Could you check a few things on this model? Use its own coordinates, in mm. A direction names the side the tool comes from. Coordinates: 2 decimals unless noted, no trailing zeros. Order: outer loops, then holes, each group sorted by start corner. A loop starts at its lowest first (then second) coordinate and runs counter-clockwise, first axis right, second up. Notation, with made-up numbers: M 88.25,18.25 L 103.25,18.25 A24 cw 103.25,57.25 Z; hole C 6.5,47.25 d9. An arc over 180 degrees is marked long. Write item = value, one per line. Start each with the question number.
from build123d import *

# Parameters (mm, degrees)
FORO_LAMATO_PER_VITE_M4_A_TESTA_CILINDRI_D           = 4.5
FORO_LAMATO_PER_VITE_M4_A_TESTA_CILINDRI_CBORE_D     = 8
FORO_LAMATO_PER_VITE_M4_A_TESTA_CILINDRI_CBORE_DEPTH = 2.6
RIPETIZIONECIRCOLARE1_COUNT                          = 4
RACCORDO1_R                                          = 1
SMUSSO1_SIZE                                         = 1
FORO_FILETTATO_M12_1_D                               = 10.2
FORO_FILETTATO_M12_1_DEPTH                           = 32.75
FORO_FILETTATO_M12_1_TIP                             = 3.064389157
SMUSSO2_SIZE                                         = 1


with BuildPart() as part:
    # Schizzo1 → Rivoluzione1 (revolve)
    with BuildSketch(Plane.XY):
        Polygon((0, 0), (0, 18.5), (8, 18.5), (8, 9), (22, 9), (22, 0), align=None)
    revolve(axis=Axis((22, 0, 0), (-1, 0, 0)))

    # Foro lamato per Vite M4 a testa cilindrica piana-1 (through all)
    with Locations(Plane.ZY):
        with Locations((0, 13)):
            foro_lamato_per_vite_m4_a_testa_cilindri = CounterBoreHole(FORO_LAMATO_PER_VITE_M4_A_TESTA_CILINDRI_D / 2, FORO_LAMATO_PER_VITE_M4_A_TESTA_CILINDRI_CBORE_D / 2, FORO_LAMATO_PER_VITE_M4_A_TESTA_CILINDRI_CBORE_DEPTH)

    # RipetizioneCircolare1: Foro lamato per Vite M4 a testa cilindrica piana-1 ×4 about axis
    ripetizionecircolare1_axis = Axis((0, 0, 0), (1, 0, 0))
    for i in range(1, RIPETIZIONECIRCOLARE1_COUNT):
        add(foro_lamato_per_vite_m4_a_testa_cilindri.rotate(ripetizionecircolare1_axis, i * 360 / RIPETIZIONECIRCOLARE1_COUNT), mode=Mode.SUBTRACT)

    # Raccordo1
    raccordo1_edges = [part.edges().sort_by_distance(p)[0] for p in [
        (8, -9, 0),
    ]]
    fillet(raccordo1_edges, radius=RACCORDO1_R)

    # Smusso1
    smusso1_edges = [part.edges().sort_by_distance(p)[0] for p in [
        (22, -9, 0),
        (8, -18.5, 0),
        (0, -18.5, 0),
    ]]
    chamfer(smusso1_edges, length=SMUSSO1_SIZE)

    # Foro filettato M12-1
    with Locations(Plane(origin=(22, 0, 0), x_dir=(0, 0, -1), z_dir=(1, 0, 0))):
        with Locations((0, 0)):
            Hole(FORO_FILETTATO_M12_1_D / 2, depth=FORO_FILETTATO_M12_1_DEPTH)
            with Locations((0, 0, -(FORO_FILETTATO_M12_1_DEPTH + FORO_FILETTATO_M12_1_TIP / 2))):  # 118° drill point
                Cone(0, FORO_FILETTATO_M12_1_D / 2, FORO_FILETTATO_M12_1_TIP, mode=Mode.SUBTRACT)

    # Smusso2
    smusso2_edges = [part.edges().sort_by_distance(p)[0] for p in [
        (0, 0, -5.1),
    ]]
    chamfer(smusso2_edges, length=SMUSSO2_SIZE)


solid = part.part
(1) Imagine slicing it at B-B on y = 0. Give the number of separate pieces and of enclosed holes in the cut face, plus the area to 3 significant figures.
(2) Will these pins go through, and if not, where does the flat tip stop? P1, Ø12, axis at x = 17.5, y = 13, coming from the -Z side; P2, Ø8, axis at x = 11, z = 4, coming from the -Y side; P3, Ø1, axis at y = -8, z = 14, coming from the -X side; P4, Ø10, axis at x = 11, z = -12.5, coming from the -Y side.
(3) Imagine slicing it at C-C on x = 14.5. List the corners of the cut face in (y, z) for me.
(4) Please list where these lines run through material, in increasing order: probe 1 along Y at (x, z) = (5.1, 0); probe 2 along Y at (x, z) = (2.15, 0); probe 3 along Z at (x, y) = (0.75, 0). Write a range as from..to.
(5) For faces 1 (the flat face through (8, 8, 8)), 2 (the flat face through (2.6, 11, 2)), 3 (the cylindrical face through (5.34, 15.23, 0.29)), which set-ups out of +Z, -Z, +X, -X, +Y, -Y let a thin tool reach every point of the face, with its end or its side?
(6) Thinking about a two-plate mould opening in Y: for faces 4 (the cylindrical face through (1.282, -0.521, -16.966)), 5 (the flat face through (22, 5, 2)), 6 (the cylindrical face through (15.084, -1.172, -8.923)), which applies, released by +Y, released by -Y, zero draft, split by the parting line, or undercut?
(7) Imagine slicing it at A-A on x = 4. List the corners of the cut face in (y, z) for me.
Response:
q1.separate_pieces = 4
q1.enclosed_holes = 0
q1.area = 230 mm2
q2.P1 = -5.66
q2.P2 = -18.14
q2.P3 = 0
q2.P4 = -15.87
q3.outline = C 0,0 d18; hole C 0,0 d10.2
q4.probe_1 = -18.5..-15.25, -10.75..-5.1, 5.1..10.75, 15.25..18.5
q4.probe_2 = -18.5..-17, -9..-5.1, 5.1..9, 17..18.5
q4.probe_3 = -18.25..-17, -9..-5.35, 5.35..9, 17..18.25
q5.face_1 = +X
q5.face_2 = -X
q5.face_3 = +X, -X
q6.face_4 = undercut
q6.face_5 = zero draft
q6.face_6 = split by the parting line
q7.outline = C 0,0 d37; hole C -13,0 d4.5; hole C 0,0 d10.2; hole C 0,-13 d4.5; hole C 0,13 d4.5; hole C 13,0 d4.5
